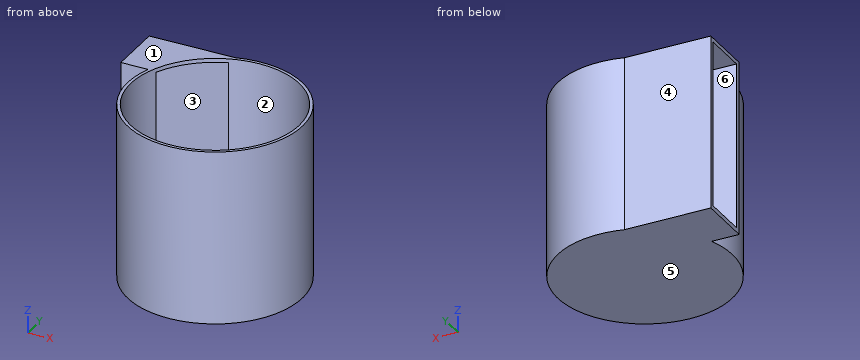
```python
from build123d import *

# Parameters (mm, degrees)
SKETCH1_R                = 105.41
BOSS_EXTRUDE1_DEPTH      = 210.82
SKETCH2_R                = 101.6
CUT_EXTRUDE1_DEPTH       = 203.2
BOSS_EXTRUDE2_DEPTH      = 203.2
BOSS_EXTRUDE2_DEPTH_BACK = 7.62
SKETCH3_W                = 132.216629509
SKETCH3_H                = 65.995330398
SKETCH4_W                = 200.799602593
SKETCH4_H                = 54.314646603
CUT_EXTRUDE2_DEPTH       = 147.574
SKETCH5_R                = 101.6
CUT_EXTRUDE3_DEPTH       = 147.574
SKETCH6_R                = 101.6
CUT_EXTRUDE4_DEPTH       = 60.706


with BuildPart() as part:
    # Sketch1 → Boss-Extrude1 (new body)
    with BuildSketch(Plane.XY):
        Circle(SKETCH1_R)
    extrude(amount=BOSS_EXTRUDE1_DEPTH)

    # Sketch2 → Cut-Extrude1 (cut)
    with BuildSketch(Plane.XY.offset(210.82)):
        Circle(SKETCH2_R)
    extrude(amount=-CUT_EXTRUDE1_DEPTH, mode=Mode.SUBTRACT)

    # Sketch3 → Boss-Extrude2 (add, two sides: drawn at the far end of the back side and taken through both)
    with BuildSketch(Plane.XY.offset(7.62).offset(-BOSS_EXTRUDE2_DEPTH_BACK)):
        with Locations((-66.108314755, 68.602334801)):
            Rectangle(SKETCH3_W, SKETCH3_H)
    extrude(amount=BOSS_EXTRUDE2_DEPTH + BOSS_EXTRUDE2_DEPTH_BACK)

    # Sketch4 → Cut-Extrude2 (cut)
    with BuildSketch(Plane.ZY.offset(132.216629509)):
        with Locations((105.657754662, 68.844414065)):
            Rectangle(SKETCH4_W, SKETCH4_H)
    extrude(amount=-CUT_EXTRUDE2_DEPTH, mode=Mode.SUBTRACT)

    # Sketch5 → Cut-Extrude3 (cut)
    with BuildSketch(Plane.XY.offset(210.82)):
        Circle(SKETCH5_R)
    extrude(amount=-CUT_EXTRUDE3_DEPTH, mode=Mode.SUBTRACT)

    # Sketch6 → Cut-Extrude4 (cut)
    with BuildSketch(Plane.XY.offset(63.246)):
        Circle(SKETCH6_R)
    extrude(amount=-CUT_EXTRUDE4_DEPTH, mode=Mode.SUBTRACT)


solid = part.part
```
Check sheet for the modelled part. Datum: model origin and axes. Units: mm. Face numbers are marked on the shaded views. A direction names the side the tool comes from. Round coordinates to 2 decimals unless told otherwise and drop trailing zeros. Order: outer loops, then holes, each group sorted by start corner. A loop starts at its lowest first (then second) coordinate and runs counter-clockwise, first axis right, second up. Notation, with made-up numbers: (57, 21.25) -> (98, 21.25) arc R26 ccw to (98, 45.25) -> close; hole circle Ø8 at (34.5, -9.5). An arc over 180 degrees is marked (long way). One line per item, written item: value. Start each with the question number.
Q1. Thickness scan on line 1 (Y direction, x = 0, z = 117); line 2 (Z direction, x = 53, y = 38.5). Record the ranges inside material, lowest first.
Q2. Cross-section at A-A (x = 0). Record the boundary of the cut face in (y, z), and give its area (3 significant figures).
Q3. Cross-section at B-B (y = 58). Record the boundary of the cut face in (x, z).
Q4. Cross-section at C-C (z = 111). Record the boundary of the cut face in (x, y), and give its area (3 significant figures).
Q5. Gauge pin test, flat ends, axial feed: pin 1 Ø10 at (x, y) = (-23, 16) entering from +Z; pin 2 Ø6 at (x, z) = (-85.5, 170) entering from +Y; pin 3 Ø2 at (y, z) = (8, 117) entering from +X. Record the tip position at first contact, or that the pin passes through.
Q6. Mould release check, pull along Z, two halves, no side actions. Record for the marked faces 4, 5 and 6: pulls with the +Z half, pulls with the -Z half, needs draft (parallel to the pull), parting line crosses it, or undercut.
Q7. Set-up check for the marked faces 1, 2 and 3: record each of +Z, -Z, +X, -X, +Y, -Y from which the full face is reachable in a straight line by a thin tool's end or side.
Completed:
1. line 1: y = -105.41 to -101.6, 101.6 to 105.41
1. line 2: z = 0 to 2.54
2. outline: (-105.41, 0) -> (105.41, 0) -> (105.41, 210.82) -> (101.6, 210.82) -> (101.6, 2.54) -> (-101.6, 2.54) -> (-101.6, 210.82) -> (-105.41, 210.82) -> close
2. area: 2,120 mm²
3. outline: (-132.22, 0) -> (88.02, 0) -> (88.02, 210.82) -> (83.42, 210.82) -> (83.42, 2.54) -> (-83.42, 2.54) -> (-83.42, 5.26) -> (-132.22, 5.26) -> close; (-132.22, 206.06) -> (-83.42, 206.06) -> (-83.42, 210.82) -> (-132.22, 210.82) -> close
4. outline: (-132.22, 35.6) -> (-99.21, 35.6) arc R105.41 ccw (long way) to (-28.08, 101.6) -> (-132.22, 101.6) -> (-132.22, 96) -> (-33.26, 96) arc R101.6 cw (long way) to (-92.65, 41.69) -> (-132.22, 41.69) -> close
4. area: 2,920 mm²
5. pin 1: stops at z = 2.54
5. pin 2: stops at y = 101.6
5. pin 3: stops at x = 105.18
6. face 4: needs draft
6. face 5: pulls with the -Z half
6. face 6: undercut
7. face 1: +Z, +X, -X, +Y, -Y
7. face 2: +Z
7. face 3: -X
